Drawing for the job (mm, zero at the part's lowest x, y, z). A direction names the side the tool comes from. Coordinates: 2 decimals unless noted, no trailing zeros. Loops run counter-clockwise (first coordinate to the right, second up) from the corner with the lowest first, then second, coordinate; pieces in that order, holes last. Notation, with made-up numbers: (-15, 6) -> (19, 6) arc R15 cw to (19, 27) -> close; hole circle Ø3 at (5, -9). An arc over 180 degrees is marked (long way). Write item = value, one per line. Start each with the question number.
(1) Drill centre lines: line 1 (Z direction, x = 17.8, y = 1.55); line 2 (X direction, y = 1.25, z = 5); line 3 (X direction, y = 0.75, z = 9.5). Where is each one in solid material? Low to high. Write a range as from..to.
(2) Band-saw the part on A-A (x = 2.2). Write the cut outline in (y, z).
(3) Band-saw the part on B-B (z = 5). Count the separate pieces of the cut face and the enclosed holes in it.
(4) Pull direction Z, two halves, no side cores. Call the marked faces 4, 5, 6 and 7: +Z half, -Z half, draft (parallel to the pull), parting line (faces both ways), or undercut.
(5) Band-saw the part on C-C (y = 7). Write the cut outline in (x, z) (1 decimal).
(6) Tool access for the marked faces 1, 2 and 3: list every direction of +Z, -Z, +X, -X, +Y, -Y with a clear straight run to the whole face (end or side of a thin tool).
(7) Flat gauge pins, fed straight in: P1, Ø1.5, axis at y = 5, z = 5.5, coming from the -X side; P2, Ø6, axis at y = 6, z = 5.5, coming from the +X side; P3, Ø1, axis at y = 3, z = 1.5, coming from the -X side; P4, Ø1.6, axis at x = 2.2, z = 5, coming from the +Y side. Where does each tip first touch, or does it go through?
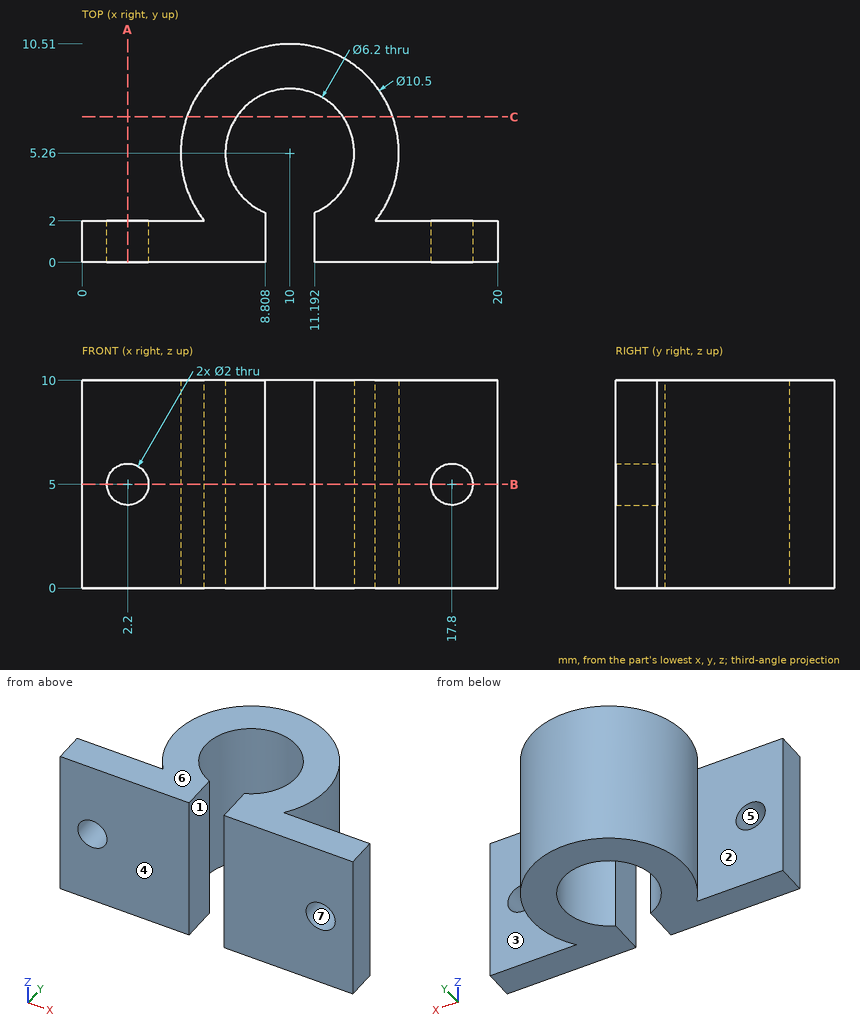
Findings below:
q1.line_1 = 0..4, 6..10
q1.line_2 = 0..1.2, 3.2..8.81, 11.19..16.8, 18.8..20
q1.line_3 = 0..8.81, 11.19..20
q2.outline = (0, 0) -> (2, 0) -> (2, 4) -> (0, 4) -> close; (0, 6) -> (2, 6) -> (2, 10) -> (0, 10) -> close
q3.separate_pieces = 3
q3.enclosed_holes = 0
q4.face_4 = draft
q4.face_5 = undercut
q4.face_6 = +Z half
q4.face_7 = undercut
q5.outline = (5, 0) -> (7.4, 0) -> (7.4, 10) -> (5, 10) -> close; (12.6, 0) -> (15, 0) -> (15, 10) -> (12.6, 10) -> close
q6.face_1 = +Z, -Z, -Y
q6.face_2 = +Z, -Z, -X
q6.face_3 = +Z, -Z, +X
q7.P1 = 4.75
q7.P2 = 15.25
q7.P3 = 5.05
q7.P4 = through
